Read the model definition and answer for the solid it produces. Units are mm, in the model's axes. A direction names the side the tool comes from. Give positions to 0.01 mm unless a question says otherwise; leave off trailing zeros. Loops run counter-clockwise (first coordinate to the right, second up) from the corner with the lowest first, then second, coordinate; pieces in that order, holes last. Notation, with made-up numbers: (81, 68.25) -> (129, 68.25) arc R16 cw to (129, 73.25) -> close; hole circle Ø2 at (-23.5, 71). An arc over 180 degrees is marked (long way). One line per item, written item: value. Start each with the question number.
from build123d import *

# Parameters (mm, degrees)
SKETCH_1_W          = 81
SKETCH_1_H          = 48
SKETCH_1_R          = 1.3
EXTRUDE_1_DEPTH     = 1
SKETCH_2_R          = 1.525
CUT_EXTRUDE_1_DEPTH = 16
SKETCH_3_W          = 55
SKETCH_3_H          = 40
CUT_EXTRUDE_2_DEPTH = 21
FILLET_1_R          = 2
SKETCH_4_W          = 20
SKETCH_4_H          = 20
EXTRUDE_2_DEPTH     = 2
FILLET_2_R          = 2
CUT_EXTRUDE_3_DEPTH = 11


with BuildPart() as part:
    # 草图1 → 凸台-拉伸1 (new, symmetric)
    with BuildSketch(Plane.XY):
        Rectangle(SKETCH_1_W, SKETCH_1_H)
        with Locations((31.5, -21)):
            Circle(SKETCH_1_R, mode=Mode.SUBTRACT)
        with Locations((-31.5, -21)):
            Circle(SKETCH_1_R, mode=Mode.SUBTRACT)
        with Locations((-31.5, 21)):
            Circle(SKETCH_1_R, mode=Mode.SUBTRACT)
        with Locations((31.5, 21)):
            Circle(SKETCH_1_R, mode=Mode.SUBTRACT)
    extrude(amount=EXTRUDE_1_DEPTH, both=True)

    # 草图2 → 切除-拉伸1 (cut, symmetric)
    with BuildSketch(Plane.XY.offset(1)):
        with Locations(Location((37.5, 21, 0), (0, 0, 180))):
            Circle(SKETCH_2_R)
        with Locations(Location((37.5, -21, 0), (0, 0, 180))):
            Circle(SKETCH_2_R)
        with Locations(Location((-37.5, -21, 0), (0, 0, 180))):
            Circle(SKETCH_2_R)
        with Locations(Location((-37.5, 21, 0), (0, 0, 180))):
            Circle(SKETCH_2_R)
    extrude(amount=CUT_EXTRUDE_1_DEPTH, both=True, mode=Mode.SUBTRACT)

    # 草图3 → 切除-拉伸2 (cut, symmetric)
    with BuildSketch(Plane.XY.offset(1)):
        Rectangle(SKETCH_3_W, SKETCH_3_H)
    extrude(amount=CUT_EXTRUDE_2_DEPTH, both=True, mode=Mode.SUBTRACT)

    # 圆角1
    fillet_1_edges = [part.edges().sort_by_distance(p)[0] for p in [
        (27.5, 20, 0),
        (27.5, -20, 0),
        (-27.5, -20, 0),
        (-27.5, 20, 0),
        (40.5, -24, 0),
        (-40.5, -24, 0),
        (-40.5, 24, 0),
        (40.5, 24, 0),
    ]]
    fillet(fillet_1_edges, radius=FILLET_1_R)

    # 草图4 → 凸台-拉伸2 (add)
    with BuildSketch(Plane(origin=(0, 0, -1), x_dir=(-1, 0, 0), z_dir=(0, 0, -1))):
        with Locations((-50.5, 0)):
            Rectangle(SKETCH_4_W, SKETCH_4_H)
    extrude(amount=-EXTRUDE_2_DEPTH)

    # 圆角2
    fillet_2_edges = [part.edges().sort_by_distance(p)[0] for p in [
        (40.5, 10, 0),
        (40.5, -10, 0),
        (60.5, -10, 0),
        (60.5, 10, 0),
    ]]
    fillet(fillet_2_edges, radius=FILLET_2_R)

    # 草图5 → 切除-拉伸3 (cut, symmetric)
    with BuildSketch(Plane.XY.offset(1)):
        with BuildLine():
            Line((32.5, 1.8), (55.5, 1.8))
            ThreePointArc((55.5, 1.8), (57.3, 0), (55.5, -1.8))
            Line((55.5, -1.8), (32.5, -1.8))
            ThreePointArc((32.5, -1.8), (30.7, 0), (32.5, 1.8))
        make_face()
        with BuildLine():
            Line((32.5, 4.2), (55.5, 4.2))
            ThreePointArc((55.5, 4.2), (57.3, 6), (55.5, 7.8))
            Line((55.5, 7.8), (32.5, 7.8))
            ThreePointArc((32.5, 7.8), (30.7, 6), (32.5, 4.2))
        make_face()
        with BuildLine():
            Line((32.5, -4.2), (55.5, -4.2))
            ThreePointArc((55.5, -4.2), (57.3, -6), (55.5, -7.8))
            Line((55.5, -7.8), (32.5, -7.8))
            ThreePointArc((32.5, -7.8), (30.7, -6), (32.5, -4.2))
        make_face()
    extrude(amount=CUT_EXTRUDE_3_DEPTH, both=True, mode=Mode.SUBTRACT)


solid = part.part
Item 1: Section C-C, the plane y = 0 is taken. Determine the outline of the cut face in (x, z).
Item 2: For faces 1 (the flat face through (51, 10, 0)), 2 (the cylindrical face through (26.9, -19.43, 0.01)), 3 (the cylindrical face through (39.9, -23.43, 0.01)), determine the directions among +Z, -Z, +X, -X, +Y, -Y from which every point of the face is accessible in a straight line to the end or side of a thin tool.
Item 3: Section B-B, the plane x = 37.5 is taken. Determine the outline of the cut face in (y, z) (3 decimals).
Item 4: Flat-ended cylindrical pins translate along their axes: pin 1 (0.6 mm diameter, centred on x = 47.5, z = 0, fed in from -Y); pin 2 (1 mm diameter, centred on y = 15.5, z = 0, fed in from +X); pin 3 (1 mm diameter, centred on x = 47.5, z = 0.5, fed in from +Y). Find the tip coordinate at first contact, or state that the pin passes through.
Item 5: Consider L1, parallel to Y at x = 33, z = 0.7; L2, parallel to Y at x = 51.5, z = 0.75; L3, parallel to Y at x = -31.5, z = 0.1. Determine where each line is inside the solid, lowest interval first. Write a range as [from, to].
Item 6: Determine the mould class of faces 4 (the cylindrical face through (41.07, -10.6, 0.01)), 5 (the flat face through (44, -4.2, 0)), 6 (the cylindrical face through (-39.93, 23.4, -0.01)) for opening direction X: pulls with the +X half, pulls with the -X half, needs draft (parallel to the pull), parting line crosses it, or undercut.
Item 7: Section D-D, the plane x = -37.5 is taken. Determine the outline of the cut face in (y, z) (3 decimals).
Item 8: Section A-A, the plane y = 21 is taken. Determine the outline of the cut face in (x, z) (3 decimals), plus the area to 3 significant figures.
Computed values:
1. outline: (-40.5, -1) -> (-27.5, -1) -> (-27.5, 1) -> (-40.5, 1) -> close; (27.5, -1) -> (30.7, -1) -> (30.7, 1) -> (27.5, 1) -> close; (57.3, -1) -> (60.5, -1) -> (60.5, 1) -> (57.3, 1) -> close
2. face 1: +Z, -Z, +X, +Y
2. face 2: +Z, -Z
2. face 3: +Z, -Z, +X, -Y
3. outline: (-24, -1) -> (-22.525, -1) -> (-22.525, 1) -> (-24, 1) -> close; (-19.475, -1) -> (-7.8, -1) -> (-7.8, 1) -> (-19.475, 1) -> close; (-4.2, -1) -> (-1.8, -1) -> (-1.8, 1) -> (-4.2, 1) -> close; (1.8, -1) -> (4.2, -1) -> (4.2, 1) -> (1.8, 1) -> close; (7.8, -1) -> (19.475, -1) -> (19.475, 1) -> (7.8, 1) -> close; (22.525, -1) -> (24, -1) -> (24, 1) -> (22.525, 1) -> close
4. pin 1: y = -10
4. pin 2: x = 40.5
4. pin 3: y = 10
5. L1: [-24, -7.8], [-4.2, -1.8], [1.8, 4.2], [7.8, 24]
5. L2: [-10, -7.8], [-4.2, -1.8], [1.8, 4.2], [7.8, 10]
5. L3: [-24, -22.3], [-19.7, 19.7], [22.3, 24]
6. face 4: pulls with the +X half
6. face 5: undercut
6. face 6: pulls with the -X half
7. outline: (-24, -1) -> (-22.525, -1) -> (-22.525, 1) -> (-24, 1) -> close; (-19.475, -1) -> (19.475, -1) -> (19.475, 1) -> (-19.475, 1) -> close; (22.525, -1) -> (24, -1) -> (24, 1) -> (22.525, 1) -> close
8. outline: (-40.5, -1) -> (-39.025, -1) -> (-39.025, 1) -> (-40.5, 1) -> close; (-35.975, -1) -> (-32.8, -1) -> (-32.8, 1) -> (-35.975, 1) -> close; (-30.2, -1) -> (30.2, -1) -> (30.2, 1) -> (-30.2, 1) -> close; (32.8, -1) -> (35.975, -1) -> (35.975, 1) -> (32.8, 1) -> close; (39.025, -1) -> (40.5, -1) -> (40.5, 1) -> (39.025, 1) -> close
8. area: 139 mm²
